Build history of the part. All positions in model axes, mm. Face numbers are marked on the shaded views. A direction names the side the tool comes from. Round coordinates to 2 decimals unless told otherwise and drop trailing zeros. Loops run counter-clockwise (first coordinate to the right, second up) from the corner with the lowest first, then second, coordinate; pieces in that order, holes last. Notation, with made-up numbers: (44.5, 67.5) - (86.5, 67.5) arc R25 ccw to (86.5, 89.5) - close; hole circle Ø6 at (21.25, -39). An arc over 180 degrees is marked (long way). Put each result on its own line as item: value. Start each with the question number.
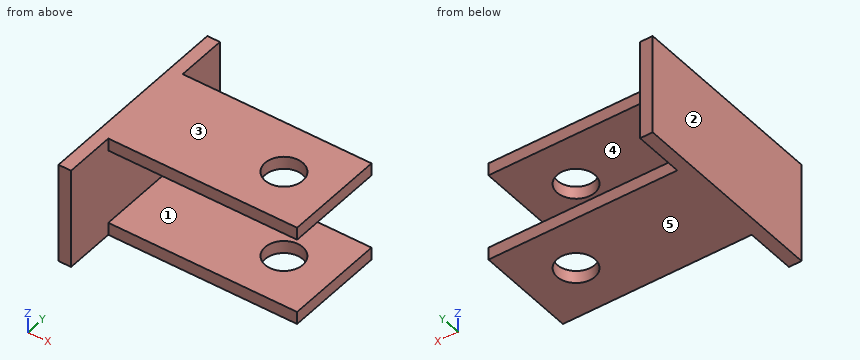
Autodesk Inventor part; units mm, degrees
ref_plane "YZ Plane" through (0, 0, 0) normal (1, 0, 0) x (0, 1, 0)
ref_plane "XZ Plane" through (0, 0, 0) normal (0, 1, 0) x (-1, 0, 0)
ref_plane "XY Plane" through (0, 0, 0) normal (0, 0, 1) x (1, 0, 0)
sketch "Sketch1" plane through (0, 0, 0) normal (0, 1, 0) x (-1, 0, 0)
  line L0 (0, 0) -> (50.8, 0)
  line L1 (50.8, 0) -> (50.8, 25.4)
  line L2 (50.8, 25.4) -> (0, 25.4)
  line L3 (0, 25.4) -> (0, 22.225)
  line L4 (0, 22.225) -> (47.625, 22.225)
  line L5 (47.625, 22.225) -> (47.625, 3.175)
  line L6 (47.625, 3.175) -> (0, 3.175)
  line L7 (0, 3.175) -> (0, 0)
  dimension "d0" = 3.175
  dimension "d1" = 3.175
  dimension "d2" = 19.05
  dimension "d3" = 50.8
extrude "Extrusion1" add sketch "Sketch1" along normal blind 25.4
sketch "Sketch2" plane through (0, 25.4, 0) normal (0, 1, 0) x (1, 0, 0)
  line L0 (-50.8, -25.4) -> (0, -25.4)
  line L1 (-50.8, -25.4) -> (-47.625, -25.4)
  line L2 (-47.625, -25.4) -> (-47.625, 0)
  line L3 (-47.625, 0) -> (-50.8, 0)
  line L4 (-50.8, 0) -> (-50.8, -25.4)
  line L5 (-47.625, -22.225) -> (-47.625, -3.175)
  line L6 (0, 0) -> (-50.8, 0)
extrude "Extrusion2" add sketch "Sketch2" along normal blind 12.7
sketch "Sketch3" plane through (0, 0, 0) normal (0, -1, 0) x (1, 0, 0)
  line L0 (-50.8, 25.4) -> (0, 25.4)
  line L1 (0, 0) -> (-47.625, 0)
  line L2 (-50.8, 25.4) -> (-47.625, 25.4)
  line L3 (-47.625, 25.4) -> (-47.625, 0)
  line L4 (-47.625, 0) -> (-50.8, 0)
  line L5 (-50.8, 0) -> (-50.8, 25.4)
extrude "Extrusion3" add sketch "Sketch3" along normal blind 12.7
sketch "Sketch4" plane through (-47.625, 0, 25.4) normal (0, 0, 1) x (1, 0, 0)
  circle A0 centre (34.925, 12.7) radius 4.7625
  line L0 (0, 0) -> (47.625, 0)
  line L1 (47.625, 0) -> (47.625, 25.4)
  dimension "d10" = 9.525
  dimension "d11" = 12.7
  dimension "d12" = 12.7
extrude "Extrusion4" cut sketch "Sketch4" against normal blind 25.4
properties part number "base" material "Aluminum 6061"
1) Drill centre lines: line 1 (Z direction, x = -38.5, y = 3) (3 decimals); line 2 (Y direction, x = -12.7, z = 24.55); line 3 (X direction, y = 28, z = 5) (3 decimals). Where is each one in solid material? Low to high. Write a range as [from, to].
2) Slice it at C-C, the plane x = -12.7. Write the cut outline in (y, z) (1 decimal).
3) Slice it at D-D, the plane z = 10.5. Write the cut outline in (x, y) (3 decimals), and give its area (3 significant figures).
4) Slice it at B-B, the plane y = 11.5. Write the cut outline in (x, z) (3 decimals).
5) Slice it at A-A, the plane x = -42.5. Write the cut outline in (y, z) (3 decimals), and give its area (3 significant figures).
6) Drop flat-ended pins along their axis: pin 1 Ø8 at (x, z) = (-18.5, 18.5) entering from -Y; pin 2 Ø10 at (x, z) = (-37.5, 21) entering from +Y; pin 3 Ø5.5 at (x, y) = (-12.7, 12.7) entering from -Z; pin 4 Ø6 at (y, z) = (9, 7) entering from +X (3 decimals). Give the stop position or say it passes through.
7) Pull direction Z, two halves, no side cores. Call the marked faces 1, 2 and 3: pulls with the +Z half, pulls with the -Z half, needs draft (parallel to the pull), parting line crosses it, or undercut.
8) Which spindle directions (+Z, -Z, +X, -X, +Y, -Y) get a long thin tool onto all of the face, cutting with end or side? Do the marked faces 4 and 5. Say none if no direction does.
Taken from the geometry:
1. line 1: z = [0, 3.175], [22.225, 25.4]
1. line 2: y = [0, 7.94], [17.46, 25.4]
1. line 3: x = [-50.8, -47.625]
2. outline: (0, 0) - (7.9, 0) - (7.9, 3.2) - (0, 3.2) - close; (0, 22.2) - (7.9, 22.2) - (7.9, 25.4) - (0, 25.4) - close; (17.5, 0) - (25.4, 0) - (25.4, 3.2) - (17.5, 3.2) - close; (17.5, 22.2) - (25.4, 22.2) - (25.4, 25.4) - (17.5, 25.4) - close
3. outline: (-50.8, -12.7) - (-47.625, -12.7) - (-47.625, 38.1) - (-50.8, 38.1) - close
3. area: 161 mm2
4. outline: (-50.8, 0) - (-17.309, 0) - (-17.309, 3.175) - (-47.625, 3.175) - (-47.625, 22.225) - (-17.309, 22.225) - (-17.309, 25.4) - (-50.8, 25.4) - close; (-8.091, 0) - (0, 0) - (0, 3.175) - (-8.091, 3.175) - close; (-8.091, 22.225) - (0, 22.225) - (0, 25.4) - (-8.091, 25.4) - close
5. outline: (0, 0) - (25.4, 0) - (25.4, 3.175) - (0, 3.175) - close; (0, 22.225) - (25.4, 22.225) - (25.4, 25.4) - (0, 25.4) - close
5. area: 161 mm2
6. pin 1: stops at y = 0
6. pin 2: stops at y = 25.4
6. pin 3: passes through
6. pin 4: stops at x = -47.625
7. face 1: undercut
7. face 2: needs draft
7. face 3: pulls with the +Z half
8. face 4: +X, +Y, -Y
8. face 5: -Z, +X, -X, +Y, -Y
